Can you work these out from the model? Positions are in its coordinate system, mm. Coordinates: 2 decimals unless noted, no trailing zeros. Order: outer loops, then holes, each group sorted by start corner. A loop starts at its lowest first (then second) coordinate and runs counter-clockwise, first axis right, second up. Notation, with made-up numbers: (-6, -8) -> (-1, -8) arc R25 cw to (-1, 26) -> close; hole circle Ø5 at (46, 57.25). An arc over 180 degrees is marked (long way). Answer in a Markdown table with one row per item. Add a question column.
1. Imagine slicing it at B-B on y = -142. Write out the boundary of the cut face in (x, z), plus the area to 3 significant figures.
2. If I drill on line 1 along Y through (x, z) = (5, 3.9); line 2 along X through (y, z) = (-142, 3.45); line 3 along X through (y, z) = (-119, 2.8), over which ranges is the centre line in solid material (lowest first)? Write a range as [from, to].
3. Will this pin go through, and if not, where does the flat tip stop? pin 1 (1.5 mm diameter, centred on x = 24, z = 2, fed in from -Y).
4. Imagine slicing it at C-C on x = 5. Write out the boundary of the cut face in (y, z).
5. Imagine slicing it at A-A on z = 2.95. Write out the boundary of the cut face in (x, y).
6. Imagine slicing it at D-D on x = 55. Write out the boundary of the cut face in (y, z).
from build123d import *

# Parameters (mm, degrees)
BOSS_EXTRU_1_DEPTH      = 5
ESQUISSE2_W             = 60
ESQUISSE2_H             = 50
BOSS_EXTRU_2_DEPTH      = 5
ESQUISSE3_R             = 2
ENL_V_MAT_EXTRU_1_DEPTH = 5


with BuildPart() as part:
    # Esquisse1 → Boss.-Extru.1 (new body)
    with BuildSketch(Plane.XY):
        Polygon((60, -50), (0, -50), (0, -150), (10, -150), (10, -100), (60, -100), align=None)
    extrude(amount=BOSS_EXTRU_1_DEPTH)

    # Esquisse2 → Boss.-Extru.2 (add)
    with BuildSketch(Plane.XY.offset(5)):
        with Locations((30, -25)):
            Rectangle(ESQUISSE2_W, ESQUISSE2_H)
    extrude(amount=-BOSS_EXTRU_2_DEPTH)

    # Esquisse3 → Enlèv. mat.-Extru.1 (cut)
    with BuildSketch(Plane.XY.offset(5)):
        with Locations((5, -142)):
            Circle(ESQUISSE3_R)
    extrude(amount=-ENL_V_MAT_EXTRU_1_DEPTH, mode=Mode.SUBTRACT)


solid = part.part
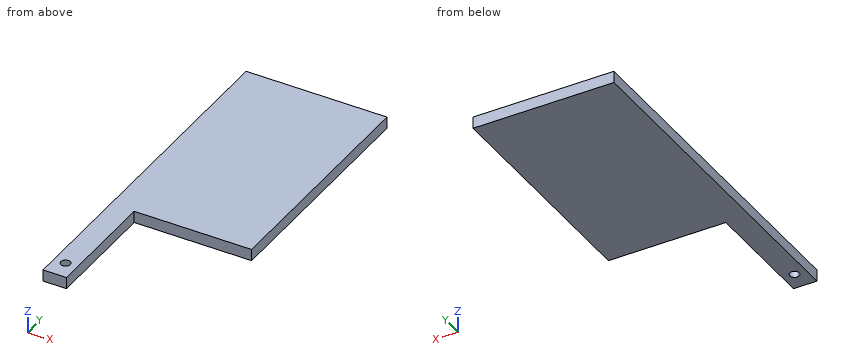
Answers follow:
| question | item | result |
|---|---|---|
| 1 | outline | (0, 0) -> (3, 0) -> (3, 5) -> (0, 5) -> close; (7, 0) -> (10, 0) -> (10, 5) -> (7, 5) -> close |
| 1 | area | 30.0 mm² |
| 2 | line 1 | y = [-150, -144], [-140, 0] |
| 2 | line 2 | x = [0, 3], [7, 10] |
| 2 | line 3 | x = [0, 10] |
| 3 | pin 1 | stops at y = -100 |
| 4 | outline | (-150, 0) -> (-144, 0) -> (-144, 5) -> (-150, 5) -> close; (-140, 0) -> (0, 0) -> (0, 5) -> (-140, 5) -> close |
| 5 | outline | (0, -150) -> (10, -150) -> (10, -100) -> (60, -100) -> (60, 0) -> (0, 0) -> close; hole circle Ø4 at (5, -142) |
| 6 | outline | (-100, 0) -> (0, 0) -> (0, 5) -> (-100, 5) -> close |
